```python
from build123d import *

# Parameters (mm, degrees)
F0_R     = 37.901352
F0_R_2   = 34.351311
F0_R_3   = 8.160883
F0_R_4   = 8.05683
F0_R_5   = 12.322845
F0_R_6   = 8.644217
F0_R_7   = 8.919641
F1_DEPTH = 25


with BuildPart() as f1:
    # F0 (on Front) → F1 (new body)
    with BuildSketch(Plane.XZ):
        Circle(F0_R)
        Circle(F0_R_2, mode=Mode.SUBTRACT)
        Circle(F0_R_2)
        with Locations((0, -22.35)):
            Circle(F0_R_3, mode=Mode.SUBTRACT)
        with Locations((-21.600001, 0)):
            Circle(F0_R_4, mode=Mode.SUBTRACT)
        Circle(F0_R_5, mode=Mode.SUBTRACT)
        with Locations((22.8, 0)):
            Circle(F0_R_6, mode=Mode.SUBTRACT)
        with Locations((0, 22.950001)):
            Circle(F0_R_7, mode=Mode.SUBTRACT)
    extrude(amount=F1_DEPTH)


solid = f1.part
```
Source: CAD feature listing. Evaluate the final solid. Frame: model axes, mm. Round coordinates to 2 decimals unless told otherwise and drop trailing zeros. Loops run counter-clockwise (first coordinate to the right, second up) from the corner with the lowest first, then second, coordinate; pieces in that order, holes last. Notation, with made-up numbers: M -3.75,-8 L 52.25,-8 A31 ccw 52.25,19 Z; hole C -20.5,-29.5 d2. An arc over 180 degrees is marked long. Use a Markdown table: item, result. Add a question column.
1. Mould query, pull axis X, two halves, no side actions, for faces 1 (the cylindrical face through (-4.93, -12.32, 37.58)), 2 (the cylindrical face through (31.045, -12.325, 2.596)), 3 (the flat face through (-9, -25, 9)). Classes: pulls with the +X half, pulls with the -X half, needs draft (parallel to the pull), parting line crosses it, or undercut.
2. Section query B-B on x = 0. Return the cut outline in (y, z).
3. Contact query for flat-ended pins moving along their axis: P1, Ø10, axis at y = -4.5, z = -10.5, coming from the -X side; P2, Ø6, axis at y = -5.5, z = 21.5, coming from the -X side; P3, Ø3, axis at y = -22, z = -27, coming from the +X side; P4, Ø12, axis at x = -19, z = 5.5, coming from the -Y side. Output: stop coordinate, or through.
4. Section query D-D on x = -16.5. Return the cut outline in (y, z).
5. Line query: line 1 (Z direction, x = 0, y = -16); line 2 (Z direction, x = -1, y = -14); line 3 (X direction, y = -16, z = -7). Output: solid intervals per line, ascending.
6. Section query A-A on z = 0. Return the cut outline in (x, y).
7. Section query C-C on z = -26.5. Return the cut outline in (x, y).
Reported:
| question | item | result |
|---|---|---|
| 1 | face 1 | parting line crosses it |
| 1 | face 2 | undercut |
| 1 | face 3 | needs draft |
| 2 | outline | M -25,-37.9 L 0,-37.9 L 0,-30.51 L -25,-30.51 Z; M -25,-14.19 L 0,-14.19 L 0,-12.32 L -25,-12.32 Z; M -25,12.32 L 0,12.32 L 0,14.03 L -25,14.03 Z; M -25,31.87 L 0,31.87 L 0,37.9 L -25,37.9 Z |
| 3 | P1 | stops at x = -37.5 |
| 3 | P2 | stops at x = -33.08 |
| 3 | P3 | stops at x = 28.04 |
| 3 | P4 | stops at y = -25 |
| 4 | outline | M -25,-34.12 L 0,-34.12 L 0,-6.24 L -25,-6.24 Z; M -25,6.24 L 0,6.24 L 0,34.12 L -25,34.12 Z |
| 5 | line 1 | z = -37.9 to -30.51, -14.19 to -12.32, 12.32 to 14.03, 31.87 to 37.9 |
| 5 | line 2 | z = -37.89 to -30.45, -14.25 to -12.28, 12.28 to 14.09, 31.81 to 37.89 |
| 5 | line 3 | x = -37.25 to -25.59, -17.61 to -10.14, 10.14 to 17.73, 27.87 to 37.25 |
| 6 | outline | M -37.9,-25 L -29.66,-25 L -29.66,0 L -37.9,0 Z; M -13.54,-25 L -12.32,-25 L -12.32,0 L -13.54,0 Z; M 12.32,-25 L 14.16,-25 L 14.16,0 L 12.32,0 Z; M 31.44,-25 L 37.9,-25 L 37.9,0 L 31.44,0 Z |
| 7 | outline | M -27.1,-25 L -7.03,-25 L -7.03,0 L -27.1,0 Z; M 7.03,-25 L 27.1,-25 L 27.1,0 L 7.03,0 Z |
